```python
from build123d import *

# Parameters (mm, degrees)
SKETCH043_R     = 1.75
SKETCH043_W     = 31.985
SKETCH043_H     = 15.1
PAD030_DEPTH    = 4
SKETCH063_R     = 1.75
POCKET011_DEPTH = 4
SKETCH076_R     = 1.75
POCKET014_DEPTH = 4
SKETCH081_R     = 1.75
POCKET016_DEPTH = 4


with BuildPart() as part:
    # Sketch043 → Pad030 (new body)
    with BuildSketch(Plane.XY):
        with BuildLine():
            Line((17.5, 50), (17.5, 78.5))
            Line((17.5, 78.5), (37.725, 78.5))
            Line((37.725, 78.5), (47.95, 78.5))
            ThreePointArc((57.95, 68.5), (55.021068, 75.571068), (47.95, 78.5))
            Line((57.95, 0), (57.95, 68.5))
            Line((57.95, -68.5), (57.95, 0))
            ThreePointArc((47.95, -78.5), (55.021068, -75.571068), (57.95, -68.5))
            Line((47.95, -78.5), (37.725, -78.5))
            Line((37.725, -78.5), (17.5, -78.5))
            Line((17.5, -50), (17.5, -78.5))
            Line((-57.5, -50), (17.5, -50))
            Line((-57.5, -50), (-57.5, -78.5))
            Line((-82.5625, -78.5), (-57.5, -78.5))
            Line((-97.625, -78.5), (-82.5625, -78.5))
            ThreePointArc((-107.625, -68.5), (-104.696068, -75.571068), (-97.625, -78.5))
            Line((-107.625, 68.500006), (-107.625, -68.5))
            ThreePointArc((-97.625, 78.5), (-104.696066, 75.57107), (-107.625, 68.500006))
            Line((-97.625, 78.5), (-82.5625, 78.5))
            Line((-57.5, 78.5), (-82.5625, 78.5))
            Line((-57.5, 50), (-57.5, 78.5))
            Line((17.5, 50), (-57.5, 50))
        make_face()
        with Locations((45.04, 60.96)):
            Circle(SKETCH043_R, mode=Mode.SUBTRACT)
        with Locations((54.96, 39.04)):
            Circle(SKETCH043_R, mode=Mode.SUBTRACT)
        with Locations((27, -42)):
            Circle(SKETCH043_R, mode=Mode.SUBTRACT)
        with Locations((12, 42)):
            Circle(SKETCH043_R, mode=Mode.SUBTRACT)
        with Locations((-57, 0)):
            Circle(SKETCH043_R, mode=Mode.SUBTRACT)
        with Locations((-20, -33.75)):
            Circle(SKETCH043_R, mode=Mode.SUBTRACT)
        with Locations((-20, -12.25)):
            Circle(SKETCH043_R, mode=Mode.SUBTRACT)
        with Locations((-20, 12.25)):
            Circle(SKETCH043_R, mode=Mode.SUBTRACT)
        with Locations((-20, 33.75)):
            Circle(SKETCH043_R, mode=Mode.SUBTRACT)
        with Locations((54.96, -39.04)):
            Circle(SKETCH043_R, mode=Mode.SUBTRACT)
        with Locations((45.04, -60.96)):
            Circle(SKETCH043_R, mode=Mode.SUBTRACT)
        with Locations((37.725, 68.5)):
            Circle(SKETCH043_R, mode=Mode.SUBTRACT)
        with Locations((47.95, 0)):
            Circle(SKETCH043_R, mode=Mode.SUBTRACT)
        with Locations((37.725, -68.5)):
            Circle(SKETCH043_R, mode=Mode.SUBTRACT)
        with Locations((-82.5625, -68.5)):
            Circle(SKETCH043_R, mode=Mode.SUBTRACT)
        with Locations((-82.5625, 68.5)):
            Circle(SKETCH043_R, mode=Mode.SUBTRACT)
        with Locations((-22.6175, 23)):
            Rectangle(SKETCH043_W, SKETCH043_H, mode=Mode.SUBTRACT)
        with Locations((-22.6175, -23)):
            Rectangle(SKETCH043_W, SKETCH043_H, mode=Mode.SUBTRACT)
    extrude(amount=PAD030_DEPTH)

    # Sketch063 → Pocket011 (cut)
    with BuildSketch(Plane(origin=(0, 0, 0), x_dir=(1, 0, 0), z_dir=(0, 0, -1))):
        with Locations((-85, 47.225)):
            Circle(SKETCH063_R)
        with Locations((-85, -46.625)):
            Circle(SKETCH063_R)
    extrude(amount=-POCKET011_DEPTH, mode=Mode.SUBTRACT)

    # Sketch076 (on Face4 of Pocket011) → Pocket014 (cut)
    with BuildSketch(Plane(origin=(0, 0, 0), x_dir=(1, 0, 0), z_dir=(0, 0, -1))):
        with Locations((40, 10)):
            Circle(SKETCH076_R)
        with Locations((40, -10)):
            Circle(SKETCH076_R)
    extrude(amount=-POCKET014_DEPTH, mode=Mode.SUBTRACT)

    # Sketch081 (on Face4 of Pocket014) → Pocket016 (cut)
    with BuildSketch(Plane(origin=(0, 0, 0), x_dir=(1, 0, 0), z_dir=(0, 0, -1))):
        with Locations((0, 20)):
            Circle(SKETCH081_R)
        with Locations((0, -20)):
            Circle(SKETCH081_R)
    extrude(amount=-POCKET016_DEPTH, mode=Mode.SUBTRACT)


solid = part.part
```
Model file for the job. Use its own axes, mm. A direction names the side the tool comes from. Coordinates: 2 decimals unless noted, no trailing zeros. Loops run counter-clockwise (first coordinate to the right, second up) from the corner with the lowest first, then second, coordinate; pieces in that order, holes last. Notation, with made-up numbers: (72, 46) - (128, 46) arc R10 ccw to (128, 58) - close; hole circle Ø8 at (79.25, 73). An arc over 180 degrees is marked (long way). Write item = value, one per line. Start each with the question number.
Item 1: Pull direction X, two halves, no side cores. Call faces 4 (the face through (-24, 1, 0)), 5 (the face through (-57.5, 64, 2)), 6 (the face through (-104.773, -75.493, 1.972)): +X half, -X half, draft (parallel to the pull), parting line (faces both ways), or undercut.
Item 2: Saw through at B-B, the plane z = 1. State how many separate pieces and enclosed holes the cut face has, then the cut area to 3 significant figures.
Item 3: Saw through at A-A, the plane y = 28.5. List the corners of the cut face in (x, z) (3 decimals).
Item 4: Drop flat-ended pins along their axis: pin 1 Ø1.5 at (x, y) = (19, -34.5) entering from -Z; pin 2 Ø1.5 at (x, z) = (-43.5, 2.5) entering from -Y; pin 3 Ø1.2 at (x, z) = (-6, 1.5) entering from +Y. Give the stop position or say it passes through.
Item 5: Wall check: probe 1 along Y at (x, z) = (45.04, 2.9); probe 2 along Y at (x, z) = (0, 3.2); probe 3 along X at (y, z) = (-50.5, 0.6) (3 decimals). Give the ranges that are in metal, low to high. Write a range as [from, to].
Item 6: 3-axis set-ups, long thin cutter, end or side, ignore diameter. For faces 1 (the face through (17.5, 64, 2)), 2 (the face through (-23, -30.55, 2)), 3 (the face through (-21, -50, 2)): which of +Z, -Z, +X, -X, +Y, -Y reach the whole face in a straight line?
Answers:
q1.face_4 = draft
q1.face_5 = undercut
q1.face_6 = -X half
q2.separate_pieces = 1
q2.enclosed_holes = 24
q2.area = 20,500 mm2
q3.outline = (-107.625, 0) - (-38.61, 0) - (-38.61, 4) - (-107.625, 4) - close; (-6.625, 0) - (57.95, 0) - (57.95, 4) - (-6.625, 4) - close
q4.pin_1 = 0
q4.pin_2 = -50
q4.pin_3 = 50
q5.probe_1 = [-78.5, -62.71], [-59.21, 59.21], [62.71, 78.5]
q5.probe_2 = [-50, -21.75], [-18.25, 18.25], [21.75, 50]
q5.probe_3 = [-107.625, -57.5], [17.5, 57.95]
q6.face_1 = +Z, -Z, +Y
q6.face_2 = +Z, -Z
q6.face_3 = +Z, -Z, -Y
